The drawing under review shows one solid part. Ordinate dimensions are in mm from its lowest x, y, z. A direction names the side the tool comes from. Coordinates: 2 decimals unless noted, no trailing zeros. Order: outer loops, then holes, each group sorted by start corner. A loop starts at its lowest first (then second) coordinate and runs counter-clockwise, first axis right, second up.
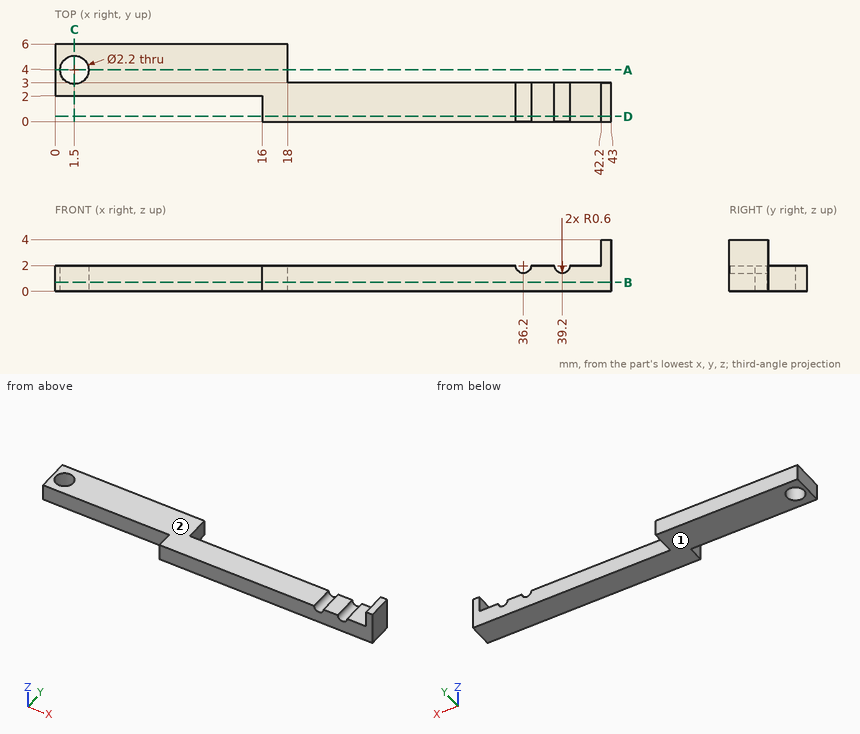
(1) Tool access review of the marked faces 1 and 2: name each direction out of +Z, -Z, +X, -X, +Y, -Y from which nothing blocks a thin tool from reaching the whole face with its end or side.
(2) Wall thickness on line 1 (X direction, y = 2.6, z = 1.95); line 2 (Y direction, x = 1.5, z = 0.6); line 3 (Y direction, x = 34.5, z = 1.6): over which ranges is each line inside the solid? List them lowest first.
(3) Consider section C-C (x = 1.5). Give the boundary of the cut face in (y, z), then the cut area to 3 significant figures.
(4) Consider section A-A (y = 4). Give the boundary of the cut face in (x, z), then the cut area to 3 significant figures.
(5) Consider section B-B (z = 0.7). Give the boundary of the cut face in (x, y).
(6) Consider section D-D (y = 0.4). Give the boundary of the cut face in (x, z), then the cut area to 3 significant figures.
(7) Insertion check: pin 1 Ø1 at (y, z) = (1.5, 3) entering from -X; pin 2 Ø1.6 at (y, z) = (4.5, 1) entering from +X; pin 3 Ø0.6 at (y, z) = (1.5, 0.5) entering from -X. Each pin has a flat end and moves straight along its axis. Give the tip position at first contact, or say it passes through.
Findings:
1. face 1: -Z, +X, -X, +Y, -Y
1. face 2: +Z, -X, +Y, -Y
2. line 1: x = 0 to 35.6, 36.8 to 38.6, 39.8 to 43
2. line 2: y = 2 to 2.9, 5.1 to 6
2. line 3: y = 0 to 3
3. outline: (2, 0) - (2.9, 0) - (2.9, 2) - (2, 2) - close; (5.1, 0) - (6, 0) - (6, 2) - (5.1, 2) - close
3. area: 3.60 mm2
4. outline: (0, 0) - (0.4, 0) - (0.4, 2) - (0, 2) - close; (2.6, 0) - (18, 0) - (18, 2) - (2.6, 2) - close
4. area: 31.6 mm2
5. outline: (0, 2) - (16, 2) - (16, 0) - (43, 0) - (43, 3) - (18, 3) - (18, 6) - (0, 6) - close; hole circle Ø2.2 at (1.5, 4)
6. outline: (16, 0) - (43, 0) - (43, 4) - (42.2, 4) - (42.2, 2) - (39.8, 2) arc R0.6 cw to (38.6, 2) - (36.8, 2) arc R0.6 cw to (35.6, 2) - (16, 2) - close
6. area: 54.5 mm2
7. pin 1: stops at x = 42.2
7. pin 2: stops at x = 18
7. pin 3: stops at x = 16
